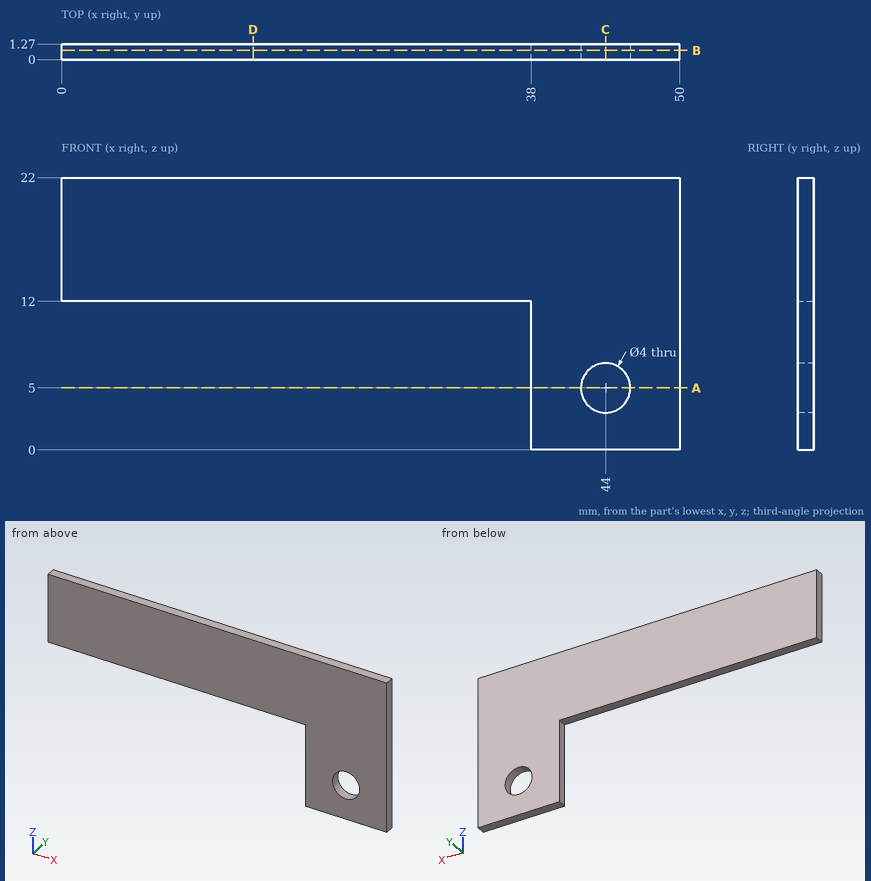
Geometry check sheet. Reference: drawing and pictorial views, mm from the part's lowest x, y, z. Coordinates: 2 decimals unless noted, no trailing zeros. Write each loop counter-clockwise with the first axis right and the second up, starting at its lowest first coordinate (ties: lowest second). Pieces come first, ordered by that corner, then holes. Notation, with made-up numbers: (-18.75, 52.5) - (16.25, 52.5) arc R12 cw to (16.25, 62.5) - close; hole circle Ø1 at (-6, 47.25). An arc over 180 degrees is marked (long way). One line per question, with ' | ' between items. Start each with the question number.
1. Material ranges on line 1 along X through (y, z) = (1.05, 5); line 2 along Z through (x, y) = (44, 0.4); line 3 along Z through (x, y) = (16, 0.75), recorded low to high.
2. Section check B-B (y = 0.75). Enter the section's corners in (x, z), plus the area to 3 significant figures.
3. Gauge pin test, flat end, axial feed: P1, Ø6, axis at x = 27.5, z = 18.5, coming from the -Y side. Record the tip position at first contact, or that the pin passes through.
4. Section check A-A (z = 5). Enter the section's corners in (x, y).
5. Section check C-C (x = 44). Enter the section's corners in (y, z).
6. Section check D-D (x = 15.5). Enter the section's corners in (y, z).
Computed values:
1) line 1: 38 to 42, 46 to 50 | line 2: 0 to 3, 7 to 22 | line 3: 12 to 22
2) outline: (0, 12) - (38, 12) - (38, 0) - (50, 0) - (50, 22) - (0, 22) - close; hole circle Ø4 at (44, 5) | area: 631 mm²
3) P1: y = 0
4) outline: (38, 0) - (42, 0) - (42, 1.27) - (38, 1.27) - close; (46, 0) - (50, 0) - (50, 1.27) - (46, 1.27) - close
5) outline: (0, 0) - (1.27, 0) - (1.27, 3) - (0, 3) - close; (0, 7) - (1.27, 7) - (1.27, 22) - (0, 22) - close
6) outline: (0, 12) - (1.27, 12) - (1.27, 22) - (0, 22) - close
